from build123d import *

# Parameters (mm, degrees)
SKETCH1_R          = 3
EXTRUDE1_DEPTH     = 8
SKETCH6_R          = 5
EXTRUDE2_DEPTH     = 6
CUT_EXTRUDE1_DEPTH = 3.75
CHAMFER1_SIZE      = 0.3


with BuildPart() as part:
    # Sketch1 → Extrude1 (new body)
    with BuildSketch(Plane.XY):
        Circle(SKETCH1_R)
    extrude(amount=-EXTRUDE1_DEPTH)

    # Sketch6 → Extrude2 (add)
    with BuildSketch(Plane(origin=(0, 0, -8), x_dir=(-1, 0, 0), z_dir=(0, 0, -1))):
        Circle(SKETCH6_R)
    extrude(amount=EXTRUDE2_DEPTH)

    # Sketch7 → Cut-Extrude1 (cut)
    with BuildSketch(Plane(origin=(0, 0, -14), x_dir=(-1, 0, 0), z_dir=(0, 0, -1))):
        Polygon((0, 2.886751346), (-2.5, 1.443375673), (-2.5, -1.443375673), (0, -2.886751346), (2.5, -1.443375673), (2.5, 1.443375673), align=None)
    extrude(amount=-CUT_EXTRUDE1_DEPTH, mode=Mode.SUBTRACT)

    # Cut-Extrude2 cone 1 section (through the dimple's axis) → Cut-Extrude2 (revolve, cut)
    with BuildSketch(Plane(origin=(0, 0, -14), x_dir=(0, 1, 0), z_dir=(1, 0, 0))):
        Polygon((0, 0), (2.886751346, 0), (0, 2.886751346), align=None)
    revolve(axis=Axis((0, 0, -14), (0, 0, 1)), mode=Mode.SUBTRACT)

    # Chamfer1
    chamfer1_edges = [part.edges().sort_by_distance(p)[0] for p in [
        (5, 0, -8),
        (5, 0, -14),
    ]]
    chamfer(chamfer1_edges, length=CHAMFER1_SIZE)

    # Sketch10 → Revolve1 (revolve)
    with BuildSketch(Plane(origin=(0, 0, 0), x_dir=(0, 0, -1), z_dir=(1, 0, 0)), mode=Mode.PRIVATE) as revolve1_sk:
        Polygon((8, 3), (8, 0), (6.507359313, 0), (7.75, 3), align=None)
    revolve(revolve1_sk.sketch.rotate(Axis((0, 0, -8), (0, 0, 1)), 270), axis=Axis((0, 0, -8), (0, 0, 1)))


solid = part.part
Verification items for the finished model (mm, model axes). A direction names the side the tool comes from. Give positions to 0.01 mm unless a question says otherwise; leave off trailing zeros. Write each loop counter-clockwise with the first axis right and the second up, starting at its lowest first coordinate (ties: lowest second). Pieces come first, ordered by that corner, then holes. Notation, with made-up numbers: M 25,24 L 42,24 A34 cw 42,60 Z; hole C -10.5,25.25 d7. An arc over 180 degrees is marked long. Write item = value, one per line.
(1) Material ranges on line 1 (Y direction, x = -4, z = -9.25); line 2 (Z direction, x = 3, y = 2); line 3 (Y direction, x = 1.25, z = -11), recorded low to high.
Found:
line_1 = -3 to 3
line_2 = -14 to -8
line_3 = -4.84 to -2.17, 2.17 to 4.84
(2) Sectioned sample at B-B (y = 0). Record the cut outline in (x, z).
Found:
outline = M -5,-13.7 L -4.7,-14 L -2.89,-14 L -2.5,-13.61 L -2.5,-10.25 L 2.5,-10.25 L 2.5,-13.61 L 2.89,-14 L 4.7,-14 L 5,-13.7 L 5,-8.3 L 4.7,-8 L 3,-8 L 3,0 L -3,0 L -3,-8 L -4.7,-8 L -5,-8.3 Z
(3) Sectioned sample at C-C (z = -5.5). Record the cut outline in (x, y), then the cut area to 3 significant figures.
Found:
outline = C 0,0 d6
area = 28.3 mm2
(4) Go/stop test with flat-tipped pins: pin 1 Ø4 at (x, z) = (-1.5, -6.5) entering from -Y; pin 2 Ø1.5 at (x, y) = (-0.5, -0.5) entering from -Z; pin 3 Ø1 at (y, z) = (-2, -2.5) entering from -X. Record where each tip stops, or that it passes through.
Found:
pin_1 = -4.96
pin_2 = -10.25
pin_3 = -2.6
(5) Access from +Z, -Z, +X, -X, +Y, -Y to the whole of each face (thin tool, end or side, straight path). Record for faces 1 (the face through (-1.36, -2.32, -13.8)), 2 (the face through (0, 0, 0)), 3 (the face through (-1, -3, -8)).
Found:
face_1 = -Z
face_2 = +Z, +X, -X, +Y, -Y
face_3 = +Z
(6) Sectioned sample at A-A (z = -11). Record the cut outline in (x, y), then the cut area to 3 significant figures.
Found:
outline = C 0,0 d10; hole M -2.5,-1.44 L 0,-2.89 L 2.5,-1.44 L 2.5,1.44 L 0,2.89 L -2.5,1.44 Z
area = 56.9 mm2
(7) Sectioned sample at D-D (z = -9.5). Record the cut outline in (x, y).
Found:
outline = C 0,0 d10
(8) Draft check along Y on faces 4 (the face through (0, 0, -10.25)), 5 (the face through (-1.268, 2.155, -12.151)), 6 (the face through (1.08, -4.88, -10.96)), 7 (the face through (0.1, -3.1, -14)). Enter one of: released by +Y, released by -Y, zero draft, split by the parting line, or undercut.
Found:
face_4 = undercut
face_5 = undercut
face_6 = split by the parting line
face_7 = zero draft
